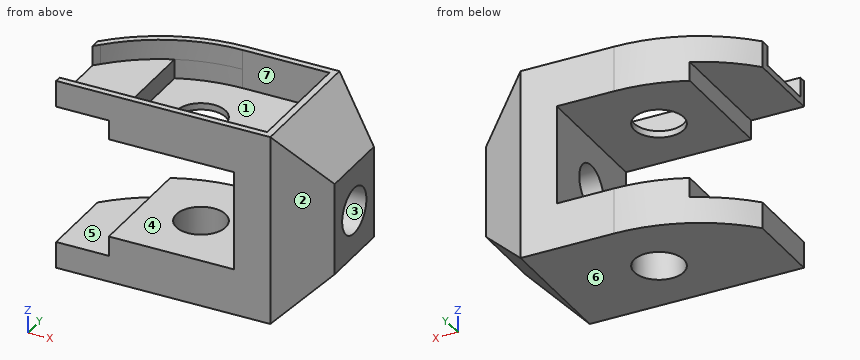
from build123d import *

# Parameters (mm, degrees)
ESQUISSE1_R              = 7.5
BOSS_EXTRU_1_DEPTH       = 58
ENL_V_MAT_EXTRU_2_DEPTH  = 107.60206377
ESQUISSE5_R              = 7
ENL_V_MAT_EXTRU_3_DEPTH  = 107.60206377
ESQUISSE11_W             = 42
ESQUISSE11_H             = 40
ENL_V_MAT_EXTRU_50_DEPTH = 16
ESQUISSE12_W             = 30.159824364
ESQUISSE12_H             = 40
ENL_V_MAT_EXTRU_51_DEPTH = 38
ENL_V_START              = -6
ESQUISSE13_R             = 7.5
ENL_V_MAT_EXTRU_52_DEPTH = 6
ENL_V_START_2            = -5.840175636
ENL_V_MAT_EXTRU_53_DEPTH = 5.840175636


with BuildPart() as part:
    # Esquisse1 → Boss.-Extru.1 (new body)
    with BuildSketch(Plane.XY):
        with BuildLine():
            Line((0, 0), (0, 24))
            Line((0, 24), (0.042431239, 24.04563747))
            ThreePointArc((0.042431239, 24.04563747), (16.689202308, 35.8382039), (36.660658521, 40))
            Line((36.660658521, 40), (65, 40))
            Line((65, 40), (80, 31.339745962))
            Line((80, 31.339745962), (80, 8.660254038))
            Line((80, 8.660254038), (65, 0))
            Line((65, 0), (0, 0))
        make_face()
        with Locations(Location((34, 19, 0), (0, 0, 180))):
            Circle(ESQUISSE1_R, mode=Mode.SUBTRACT)
    extrude(amount=BOSS_EXTRU_1_DEPTH)

    # Esquisse4 → Enlèv. mat.-Extru.2 (cut, through all)
    with BuildSketch(Plane.XZ):
        Polygon((65, 58), (80, 43), (80, 58), align=None)
        Polygon((65, 0), (80, 0), (80, 15), align=None)
    extrude(amount=-ENL_V_MAT_EXTRU_2_DEPTH, mode=Mode.SUBTRACT)

    # Esquisse5 → Enlèv. mat.-Extru.3 (cut, through all)
    with BuildSketch(Plane(origin=(80, 0, 0), x_dir=(0, 0, -1), z_dir=(1, 0, 0))):
        with Locations((-29, 20)):
            Circle(ESQUISSE5_R)
    extrude(amount=-ENL_V_MAT_EXTRU_3_DEPTH, mode=Mode.SUBTRACT)

    # Esquisse11 → Enlèv. mat.-Extru.50 (cut)
    with BuildSketch(Plane.ZY):
        with Locations((29, 20)):
            Rectangle(ESQUISSE11_W, ESQUISSE11_H)
    extrude(amount=-ENL_V_MAT_EXTRU_50_DEPTH, mode=Mode.SUBTRACT)

    # Esquisse12 → Enlèv. mat.-Extru.51 (cut)
    with BuildSketch(Plane.ZY.offset(-16)):
        with Locations((29.079912182, 20)):
            Rectangle(ESQUISSE12_W, ESQUISSE12_H)
    extrude(amount=-ENL_V_MAT_EXTRU_51_DEPTH, mode=Mode.SUBTRACT)

    # Esquisse13 → Enlèv. mat.-Extru.52 (cut)
    with BuildSketch(Plane.XY.offset(58).offset(ENL_V_START)):
        with BuildLine():
            Line((0, 21.176651641), (0, 2))
            Line((0, 2), (63, 2))
            Line((63, 2), (63, 38))
            Line((63, 38), (36.660658521, 38))
            ThreePointArc((36.660658521, 38), (17.488060557, 34.004675744), (1.507160331, 22.683811971))
            Line((1.507160331, 22.683811971), (0, 21.176651641))
        make_face()
        with Locations(Location((34, 19, 0), (0, 0, 180))):
            Circle(ESQUISSE13_R, mode=Mode.SUBTRACT)
    extrude(amount=ENL_V_MAT_EXTRU_52_DEPTH, mode=Mode.SUBTRACT)

    # Esquisse14 → Enlèv. mat.-Extru.53 (cut)
    with BuildSketch(Plane.XY.offset(52).offset(ENL_V_START_2)):
        with BuildLine():
            Line((63, 38), (63, 2))
            Line((63, 2), (18, 2))
            Line((18, 2), (18, 34.224199524))
            ThreePointArc((18, 34.224199524), (27.141246175, 37.046581051), (36.660658521, 38))
            Line((36.660658521, 38), (63, 38))
        make_face()
    extrude(amount=ENL_V_MAT_EXTRU_53_DEPTH, mode=Mode.SUBTRACT)


solid = part.part
The model under review builds one solid part; all positions refer to its coordinate system, in mm. Face numbers are marked on the shaded views. A direction names the side the tool comes from. Coordinates: 2 decimals unless noted, no trailing zeros. Loops run counter-clockwise (first coordinate to the right, second up) from the corner with the lowest first, then second, coordinate; pieces in that order, holes last.
(1) Wall thickness on L1, parallel to Z at x = 51.5, y = 37; L2, parallel to Z at x = 8, y = 7; L3, parallel to X at y = 22.5, z = 42.5: over which ranges is each line inside the solid? List them lowest first.
Determined:
L1: z = 0 to 14, 44.16 to 46.16
L2: z = 0 to 8, 50 to 52
L3: x = 54 to 80
(2) Consider section A-A, the plane z = 29. Give the boundary of the cut face in (x, y), plus the area to 3 significant figures.
Determined:
outline: (54, 0) - (65, 0) - (80, 8.66) - (80, 13) - (54, 13) - close; (54, 27) - (80, 27) - (80, 31.34) - (65, 40) - (54, 40) - close
area: 546 mm2
(3) Insertion check: P1, Ø1.5, axis at y = 13, z = 36, coming from the -X side; P2, Ø1, axis at y = 25, z = 25.5, coming from the +X side; P3, Ø3, axis at y = 26, z = 11, coming from the -X side; P4, Ø11, axis at x = 35.5, y = 24, coming from the +Z side. Each pin has a flat end and moves straight along its axis. Give the tip position at first contact, or say it passes through.
Determined:
P1: stops at x = 54
P2: passes through
P3: stops at x = 16
P4: stops at z = 46.16
(4) Draft analysis for pull direction Y (two halves, no side actions). For the marked faces 1, 2, 3 and 4, state which applies: +Y half, -Y half, draft (parallel to the pull), parting line (faces both ways), or undercut.
Determined:
face 1: undercut
face 2: -Y half
face 3: undercut
face 4: draft
(5) Consider section D-D, the plane z = 6.5. Give the boundary of the cut face in (x, y).
Determined:
outline: (0, 0) - (65, 0) - (71.5, 3.75) - (71.5, 36.25) - (65, 40) - (36.66, 40) arc R50 ccw to (0.04, 24.05) - (0, 24) - close; hole circle Ø15 at (34, 19)
(6) Tool access review of the marked faces 5, 6 and 7: name each direction out of +Z, -Z, +X, -X, +Y, -Y from which nothing blocks a thin tool from reaching the whole face with its end or side.
Determined:
face 5: -X, +Y, -Y
face 6: -Z, +X, -X, +Y, -Y
face 7: +Z
(7) Consider section C-C, the plane x = 34. Give the boundary of the cut face in (y, z).
Determined:
outline: (0, 0) - (11.5, 0) - (11.5, 14) - (0, 14) - close; (0, 44.16) - (11.5, 44.16) - (11.5, 46.16) - (2, 46.16) - (2, 58) - (0, 58) - close; (26.5, 0) - (39.93, 0) - (39.93, 14) - (26.5, 14) - close; (26.5, 44.16) - (39.93, 44.16) - (39.93, 58) - (37.93, 58) - (37.93, 46.16) - (26.5, 46.16) - close
(8) Consider section B-B, the plane y = 20. Give the number of separate pieces and of enclosed holes in the cut face, plus the area to 3 significant figures.
Determined:
separate pieces: 4
enclosed holes: 0
area: 1,350 mm2
